from build123d import *

# Parameters (mm, degrees)
EXTRUDE_1_DEPTH          = 2
EXTRUDE_2_DEPTH          = 3
SKETCH_3_W               = 16
SKETCH_3_H               = 60
EXTRUDE_3_DEPTH          = 3
CUT_EXTRUDE_1_DEPTH      = 1
CUT_EXTRUDE_2_DEPTH      = 69.543781629
SKETCH_6_W               = 20
SKETCH_6_H               = 16.5
CUT_EXTRUDE_4_DEPTH      = 2
CUT_EXTRUDE_6_DEPTH      = 69.543781629
CUT_EXTRUDE_6_DEPTH_BACK = 69.543781629
EXTRUDE_START            = -1
EXTRUDE_4_DEPTH          = 1
SKETCH_12_R              = 1
SKETCH_12_R_2            = 4
CUT_EXTRUDE_7_DEPTH      = 2.54
SKETCH_13_R              = 1.25
CUT_EXTRUDE_8_DEPTH      = 10
SKETCH_15_R              = 1
CUT_EXTRUDE_10_DEPTH     = 10
SKETCH_16_R              = 1.02
CUT_EXTRUDE_11_DEPTH     = 2
SKETCH_19_R              = 1.808389453
SKETCH_19_R_2            = 1.798107518
SKETCH_19_R_3            = 1.231148897
SKETCH_19_R_4            = 1.358627773
EXTRUDE_5_DEPTH          = 2
EXTRUDE_START_2          = -3
SKETCH_19_3_R            = 1.231148897
SKETCH_19_3_R_2          = 1.358627773
EXTRUDE_6_DEPTH          = 1
HOLE_WIZARD_M2_5_1_D     = 2.05
HOLE_WIZARD_M2_1_D       = 1.6
SKETCH_25_R              = 4.02
CUT_EXTRUDE_12_DEPTH     = 2.54
SKETCH_30_W              = 55.306598362
SKETCH_30_H              = 0.5
CUT_EXTRUDE_17_DEPTH     = 75.310646225
SKETCH_31_W              = 47.74998635
SKETCH_31_H              = 36.890870636
CUT_EXTRUDE_18_DEPTH     = 75.22986018
SKETCH_32_W              = 16
SKETCH_32_H              = 6
CUT_EXTRUDE_19_DEPTH     = 2
FILLET_2_R               = 2
SKETCH_33_R              = 1.25
CUT_EXTRUDE_20_DEPTH     = 2
SKETCH_35_R              = 4.02
EXTRUDE_7_DEPTH          = 4
SKETCH_36_R              = 4.04
CUT_EXTRUDE_21_DEPTH     = 2.54
SKETCH_37_W              = 31
SKETCH_37_H              = 0.5
CUT_EXTRUDE_22_DEPTH     = 10
SKETCH_38_R              = 1.3
CUT_EXTRUDE_23_DEPTH     = 44.324358045


with BuildPart() as part:
    # 草图1 → 凸台-拉伸1 (new body)
    with BuildSketch(Plane(origin=(0, 0, 0), x_dir=(1, 0, 0), z_dir=(0, 1, 0))):
        with BuildLine():
            Line((43, 1.5), (58.456841673, 3.534931811))
            ThreePointArc((58.456841673, 3.534931811), (61.401458892, 6.180320766), (59.995303837, 9.880534443))
            Line((59.995303837, 9.880534443), (31, 30))
            Line((31, 30), (10, 30))
            Line((10, 30), (0, 15))
            Line((0, 15), (0, -15))
            Line((0, -15), (10, -30))
            Line((10, -30), (31, -30))
            Line((31, -30), (59.995303837, -9.880534443))
            ThreePointArc((59.995303837, -9.880534443), (61.401458892, -6.180320766), (58.456841673, -3.534931811))
            Line((58.456841673, -3.534931811), (43, -1.5))
            Line((43, -1.5), (40, -1.5))
            Line((40, -1.5), (40, 1.5))
            Line((40, 1.5), (43, 1.5))
        make_face()
    extrude(amount=EXTRUDE_1_DEPTH)

    # 草图2 → 凸台-拉伸2 (add)
    with BuildSketch(Plane.XZ):
        Polygon((15, -30), (15, 30), (10, 30), (0, 15), (0, -15), (10, -30), align=None)
    extrude(amount=EXTRUDE_2_DEPTH)

    # 草图3 → 凸台-拉伸3 (add)
    with BuildSketch(Plane.XZ):
        with Locations((23, 0)):
            Rectangle(SKETCH_3_W, SKETCH_3_H)
    extrude(amount=EXTRUDE_3_DEPTH)

    # 草图5 → 切除-拉伸1 (cut)
    with BuildSketch(Plane.XZ.offset(3)):
        Polygon((10, -30), (31, -30), (31, 30), (10, 30), (0, 15), (0, -15), align=None)
    extrude(amount=-CUT_EXTRUDE_1_DEPTH, mode=Mode.SUBTRACT)

    # 草图4 → 切除-拉伸2 (cut, through all)
    with BuildSketch(Plane(origin=(0, 2, 0), x_dir=(1, 0, 0), z_dir=(0, 1, 0))):
        Polygon((15, -30.054194631), (25, -30), (25, -13.5), (15, -13.5), align=None)
        Polygon((25, 13.5), (15, 13.5), (15, 30.054194631), (25, 30), align=None)
    extrude(amount=-CUT_EXTRUDE_2_DEPTH, mode=Mode.SUBTRACT)

    # 草图6 → 切除-拉伸4 (cut)
    with BuildSketch(Plane(origin=(0, 2, 0), x_dir=(1, 0, 0), z_dir=(0, 1, 0))):
        with Locations((20, 21.75)):
            Rectangle(SKETCH_6_W, SKETCH_6_H)
        with Locations((20, -21.75)):
            Rectangle(SKETCH_6_W, SKETCH_6_H)
    extrude(amount=-CUT_EXTRUDE_4_DEPTH, mode=Mode.SUBTRACT)

    # 草图10 → 切除-拉伸6 (cut, two sides: drawn at the far end of the back side and taken through both)
    with BuildSketch(Plane(origin=(0, 2, 0), x_dir=(1, 0, 0), z_dir=(0, 1, 0)).offset(-CUT_EXTRUDE_6_DEPTH_BACK)):
        Polygon((40, -1.5), (-11.100796723, -1.5), (-3.854090755, 32.230988753), (54.203821011, 29.618804043), (85.46449539, 13.041941672), (77.376427304, 2.654316721), align=None)
    extrude(amount=CUT_EXTRUDE_6_DEPTH + CUT_EXTRUDE_6_DEPTH_BACK, mode=Mode.SUBTRACT)

    # 草图11 → 凸台-拉伸4 (add)
    with BuildSketch(Plane(origin=(0, 2, 0), x_dir=(1, 0, 0), z_dir=(0, 1, 0)).offset(EXTRUDE_START)):
        with BuildLine():
            Line((31, -34.868641247), (62.27565108, -13.166872292))
            ThreePointArc((62.27565108, -13.166872292), (65.15434027, -9.255636577), (65.033342884, -4.400744621))
            Line((65.033342884, -4.400744621), (58.456841673, -3.534931811))
            ThreePointArc((58.456841673, -3.534931811), (61.401458892, -6.180320766), (59.995303837, -9.880534443))
            Line((59.995303837, -9.880534443), (31, -30))
            Line((31, -30), (31, -34))
            Line((31, -34), (31, -34.868641247))
        make_face()
    extrude(amount=EXTRUDE_4_DEPTH)

    # 草图12 → 切除-拉伸7 (cut)
    with BuildSketch(Plane(origin=(0, 2, 0), x_dir=(1, 0, 0), z_dir=(0, 1, 0))):
        with Locations(Location((58, -7.004988826, 0), (0, 0, 270))):
            Circle(SKETCH_12_R)
        with Locations(Location((43, -6, 0), (0, 0, 270))):
            Circle(SKETCH_12_R)
        with Locations(Location((6, -7.25, 0), (0, 0, 270))):
            Circle(SKETCH_12_R_2)
    extrude(amount=-CUT_EXTRUDE_7_DEPTH, mode=Mode.SUBTRACT)

    # 草图13 → 切除-拉伸8 (cut)
    with BuildSketch(Plane(origin=(0, 0, 0), x_dir=(1, 0, 0), z_dir=(0, 1, 0))):
        with Locations(Location((13, -21.75, 0), (0, 0, 270))):
            Circle(SKETCH_13_R)
        with Locations(Location((27, -21.75, 0), (0, 0, 270))):
            Circle(SKETCH_13_R)
    extrude(amount=-CUT_EXTRUDE_8_DEPTH, mode=Mode.SUBTRACT)

    # 草图15 → 切除-拉伸10 (cut)
    with BuildSketch(Plane.XZ.offset(-1)):
        with Locations(Location((36, 29.573465579, 0), (0, 0, 270))):
            Circle(SKETCH_15_R)
        with Locations(Location((56, 15.695724776, 0), (0, 0, 270))):
            Circle(SKETCH_15_R)
    extrude(amount=-CUT_EXTRUDE_10_DEPTH, mode=Mode.SUBTRACT)

    # 草图16 → 切除-拉伸11 (cut)
    with BuildSketch(Plane.XZ):
        with Locations(Location((58, 7.004988826, 0), (0, 0, 270))):
            Circle(SKETCH_16_R)
        with Locations(Location((43, 6, 0), (0, 0, 270))):
            Circle(SKETCH_16_R)
    extrude(amount=-CUT_EXTRUDE_11_DEPTH, mode=Mode.SUBTRACT)

    # 草图19 → 凸台-拉伸5 (add)
    with BuildSketch(Plane.XZ.offset(2)):
        with Locations((13, 21.75)):
            Circle(SKETCH_19_R)
        with Locations((27, 21.75)):
            Circle(SKETCH_19_R_2)
        with Locations((36, 29.573465579)):
            Circle(SKETCH_19_R_3)
        with Locations((56, 15.695724776)):
            Circle(SKETCH_19_R_4)
    extrude(amount=-EXTRUDE_5_DEPTH)


with BuildPart() as extrude_5_kept_piece:
    # of the separate pieces the step leaves, the one the design keeps (extrude_5_pieces_kept)
    add(part.part.solids().sort_by_distance((58.456841673, 0, 3.534931811))[0])

    # 草图19<3> → 凸台-拉伸6 (add)
    with BuildSketch(Plane.XZ.offset(2).offset(EXTRUDE_START_2)):
        with Locations((36, 29.573465579)):
            Circle(SKETCH_19_3_R)
        with Locations((56, 15.695724776)):
            Circle(SKETCH_19_3_R_2)
    extrude(amount=-EXTRUDE_6_DEPTH)

    # M2.5 螺纹孔1 (through all)
    with Locations(Plane(origin=(0, -2, 0), x_dir=(-1, 0, 0), z_dir=(0, -1, 0))):
        with Locations((-27, -21.75), (-13, -21.75)):
            Hole(HOLE_WIZARD_M2_5_1_D / 2)

    # M2 螺纹孔1 (through all)
    with Locations(Plane(origin=(0, 1, 0), x_dir=(-1, 0, 0), z_dir=(0, -1, 0))):
        with Locations((-56, -15.695724776), (-36, -29.573465579)):
            Hole(HOLE_WIZARD_M2_1_D / 2)

    # 草图25 → 切除-拉伸12 (cut)
    with BuildSketch(Plane(origin=(0, 2, 0), x_dir=(1, 0, 0), z_dir=(0, 1, 0))):
        with Locations(Location((6, -7.25, 0), (0, 0, 270))):
            Circle(SKETCH_25_R)
    extrude(amount=-CUT_EXTRUDE_12_DEPTH, mode=Mode.SUBTRACT)

    # 草图30 → 切除-拉伸17 (cut, through all)
    with BuildSketch(Plane.XZ.offset(2)):
        with Locations((27.653299181, 1.75)):
            Rectangle(SKETCH_30_W, SKETCH_30_H)
    extrude(amount=-CUT_EXTRUDE_17_DEPTH, mode=Mode.SUBTRACT)

    # 草图31 → 切除-拉伸18 (cut, through all)
    with BuildSketch(Plane.XZ):
        with Locations((54.874993175, 20.445435318)):
            Rectangle(SKETCH_31_W, SKETCH_31_H)
    extrude(amount=-CUT_EXTRUDE_18_DEPTH, mode=Mode.SUBTRACT)

    # 草图32 → 切除-拉伸19 (cut)
    with BuildSketch(Plane(origin=(0, 2, 0), x_dir=(1, 0, 0), z_dir=(0, 1, 0))):
        with Locations((23, -8)):
            Rectangle(SKETCH_32_W, SKETCH_32_H)
    extrude(amount=-CUT_EXTRUDE_19_DEPTH, mode=Mode.SUBTRACT)

    # 圆角2
    fillet_2_edges = [extrude_5_kept_piece.edges().sort_by_distance(p)[0] for p in [
        (31, 1, 5),
        (31, 1, 11),
        (15, 1, 11),
        (15, 1, 5),
    ]]
    fillet(fillet_2_edges, radius=FILLET_2_R)

    # 草图33 → 切除-拉伸20 (cut)
    with BuildSketch(Plane(origin=(0, 0, 0), x_dir=(1, 0, 0), z_dir=(0, 1, 0))):
        with Locations(Location((19, -8, 0), (0, 0, 270))):
            Circle(SKETCH_33_R)
        with Locations(Location((23.5, -8, 0), (0, 0, 270))):
            Circle(SKETCH_33_R)
        with Locations(Location((28, -8, 0), (0, 0, 270))):
            Circle(SKETCH_33_R)
    extrude(amount=-CUT_EXTRUDE_20_DEPTH, mode=Mode.SUBTRACT)

    # 草图35 → 凸台-拉伸7 (add)
    with BuildSketch(Plane(origin=(0, 2, 0), x_dir=(1, 0, 0), z_dir=(0, 1, 0))):
        with Locations((6, -7.25)):
            Circle(SKETCH_35_R)
    extrude(amount=-EXTRUDE_7_DEPTH)

    # 草图36 → 切除-拉伸21 (cut)
    with BuildSketch(Plane(origin=(0, 2, 0), x_dir=(1, 0, 0), z_dir=(0, 1, 0))):
        with Locations(Location((6, -7.5, 0), (0, 0, 270))):
            Circle(SKETCH_36_R)
    extrude(amount=-CUT_EXTRUDE_21_DEPTH, mode=Mode.SUBTRACT)

    # 草图37 → 切除-拉伸22 (cut)
    with BuildSketch(Plane(origin=(0, 2, 0), x_dir=(1, 0, 0), z_dir=(0, 1, 0))):
        with Locations((15.5, -2.25)):
            Rectangle(SKETCH_37_W, SKETCH_37_H)
    extrude(amount=-CUT_EXTRUDE_22_DEPTH, mode=Mode.SUBTRACT)

    # 草图38 → 切除-拉伸23 (cut, through all)
    with BuildSketch(Plane.XZ.offset(2)):
        with Locations(Location((19, 8, 0), (0, 0, 270))):
            Circle(SKETCH_38_R)
    extrude(amount=-CUT_EXTRUDE_23_DEPTH, mode=Mode.SUBTRACT)


solid = extrude_5_kept_piece.part
Source: CAD feature listing. Evaluate the final solid. Frame: model axes, mm. A direction names the side the tool comes from. Give positions to 0.01 mm unless a question says otherwise; leave off trailing zeros. Write each loop counter-clockwise with the first axis right and the second up, starting at its lowest first coordinate (ties: lowest second). Pieces come first, ordered by that corner, then holes. Notation, with made-up numbers: M 2.25,6 L 21.25,6 A27 cw 21.25,38 Z; hole C -8,73.25 d5. An arc over 180 degrees is marked long. Return JSON: item names as keys, results as strings. Group by question number.
1) Set-up query: faces 1 (the face through (30, 1, 22)), 2 (the face through (15, -1, 22)), 3 (the face through (15.6, 0.99, 5.57)). Return all of +Z, -Z, +X, -X, +Y, -Y with unobstructed straight access to the full face (end or side cutting, diameter ignored); none if empty.
2) Cut plane D-D, the plane x = 6. Output: boundary loops of the cut face in (y, z), plus the area to 3 significant figures.
3) Pull-direction query (X, two-part tool) for faces 4 (the face through (15.57, 0.99, 10.4)), 5 (the face through (13, 2, 12)), 6 (the face through (29, 0, 22)); classes: pulls with the +X half, pulls with the -X half, needs draft (parallel to the pull), parting line crosses it, or undercut.
4) Cut plane C-C, the plane y = 1.15. Output: boundary loops of the cut face in (x, z).
5) Cut plane A-A, the plane x = 23.5. Output: boundary loops of the cut face in (y, z), plus the area to 3 significant figures.
6) Material intervals for line 1 along X through (y, z) = (-1.1, 8); line 2 along X through (y, z) = (-1.2, 18); line 3 along X through (y, z) = (-0.75, 28.5), sorted ascending. Write a range as [from, to].
7) Cut plane B-B, the plane z = 21.75. Output: boundary loops of the cut face in (x, y) (3 decimals).
8) Pin query (flat end, axial travel): P1, Ø1.6, axis at x = 21, y = 0.5, coming from the +Z side; P2, Ø2, axis at y = -1.5, z = 22, coming from the -X side; P3, Ø2.5, axis at x = 13, z = 21.75, coming from the -Y side; P4, Ø4, axis at x = 19, z = 8, coming from the +Y side. Return the tip coordinate at first contact, or that it passes through.
Recorded:
{
 "1": {"face 1": "+Z, +Y", "face 2": "+Z, +Y, -Y", "face 3": "+X, +Y"},
 "2": {"outline": "M -2,2.5 L 2,2.5 L 2,3.46 L -0.54,3.46 L -0.54,11.54 L 2,11.54 L 2,24 L -2,24 Z", "area": "65.5 mm²"},
 "3": {"face 4": "pulls with the +X half", "face 5": "needs draft", "face 6": "undercut"},
 "4": {"outline": "M 0,2.5 L 31,2.5 L 31,3 A2 ccw 29,5 L 17,5 A2 cw 15,7 L 15,9 A2 cw 17,11 L 29,11 A2 ccw 31,13 L 31,30 L 30,30 L 30,13.5 L 10,13.5 L 10,30 L 0,15 Z; hole C 6,7.5 d8.08"},
 "5": {"outline": "M -2,2.5 L 2,2.5 L 2,5 L 0,5 L 0,6.75 L -2,6.75 Z; M -2,9.25 L 0,9.25 L 0,11 L 2,11 L 2,13.5 L -2,13.5 Z", "area": "27.0 mm²"},
 "6": {"line 1": "x = [0, 17.7], [20.3, 22.25], [24.75, 26.75], [29.25, 31]", "line 2": "x = [2, 15], [25, 31]", "line 3": "x = [9, 15], [25, 31]"},
 "7": {"outline": "M 4.5,-2 L 11.975,-2 L 11.975,0 L 10,0 L 10,2 L 4.5,2 Z; M 14.025,-2 L 15,-2 L 15,0 L 14.025,0 Z; M 25,-2 L 25.975,-2 L 25.975,0 L 25,0 Z; M 28.025,-2 L 31,-2 L 31,2 L 30,2 L 30,0 L 28.025,0 Z"},
 "8": {"P1": "stops at z = 13.5", "P2": "stops at x = 4", "P3": "stops at y = -2", "P4": "stops at y = 0"}
}
